For this review, take the finished solid that the model builds, in its own axes (mm). Face numbers are marked on the shaded views. A direction names the side the tool comes from. Round coordinates to 2 decimals unless told otherwise and drop trailing zeros. Order: outer loops, then holes, each group sorted by start corner. A loop starts at its lowest first (then second) coordinate and runs counter-clockwise, first axis right, second up. Notation, with made-up numbers: (-3.5, 54) -> (14.5, 54) arc R6 ccw to (14.5, 60) -> close; hole circle Ø1 at (12, 80.5). An arc over 180 degrees is marked (long way). Answer in a Markdown table with one row per item.
```python
from build123d import *

# Parameters (mm, degrees)
SKETCH1_W           = 300
SKETCH1_H           = 300
BOSS_EXTRUDE1_DEPTH = 120
SKETCH3_R           = 17.5
BOSS_EXTRUDE3_DEPTH = 60
FILLET1_R           = 5
SKETCH4_R           = 51
BOSS_EXTRUDE4_DEPTH = 50
FILLET2_R           = 50
SKETCH6_R           = 7.5
BOSS_EXTRUDE5_DEPTH = 20


with BuildPart() as part:
    # Sketch1 → Boss-Extrude1 (new body)
    with BuildSketch(Plane(origin=(0, 0, 0), x_dir=(1, 0, 0), z_dir=(0, 1, 0))):
        Rectangle(SKETCH1_W, SKETCH1_H)
    extrude(amount=BOSS_EXTRUDE1_DEPTH)

    # Sketch3 → Boss-Extrude3 (add)
    with BuildSketch(Plane.XY.offset(150)):
        with Locations(Location((-115, 25, 0), (0, 0, 180))):
            Circle(SKETCH3_R)
    boss_extrude3 = extrude(amount=BOSS_EXTRUDE3_DEPTH)

    # Mirror1: Boss-Extrude3 across plane
    add(boss_extrude3.mirror(Plane.XY))

    # Fillet1
    fillet1_edges = [part.edges().sort_by_distance(p)[0] for p in [
        (-97.5, 25, 150),
        (-97.5, 25, -150),
    ]]
    fillet(fillet1_edges, radius=FILLET1_R)

    # Sketch4 → Boss-Extrude4 (add)
    with BuildSketch(Plane.XZ):
        with Locations(Location((90, 0, 0), (0, 0, 90))):
            Circle(SKETCH4_R)
    extrude(amount=BOSS_EXTRUDE4_DEPTH)

    # Fillet2
    fillet2_edges = [part.edges().sort_by_distance(p)[0] for p in [
        (90, -50, -51),
    ]]
    fillet(fillet2_edges, radius=FILLET2_R - 0.0001)  # a hair under: the kernel refuses the full size

    # Sketch6 → Boss-Extrude5 (add)
    with BuildSketch(Plane(origin=(150, 0, 0), x_dir=(0, 0, -1), z_dir=(1, 0, 0))):
        with Locations(Location((-75, 50, 0), (0, 0, 180))):
            Circle(SKETCH6_R)
        with Locations(Location((75, 50, 0), (0, 0, 180))):
            Circle(SKETCH6_R)
    extrude(amount=BOSS_EXTRUDE5_DEPTH)


solid = part.part
```
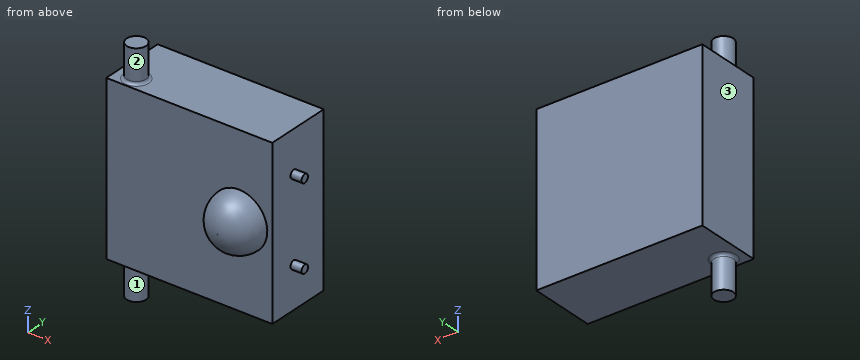
Q1. Take a section at A-A, the plane z = -75. Write out the cut boundary in (x, y).
Answer key:
| item | result |
|---|---|
| outline | (-150, 0) -> (150, 0) -> (150, 42.5) -> (170, 42.5) -> (170, 57.5) -> (150, 57.5) -> (150, 120) -> (-150, 120) -> close |
Q2. Take a section at B-B, the plane x = -115. Write out the cut boundary in (y, z), then the cut area to 3 significant figures.
Answer key:
| item | result |
|---|---|
| outline | (0, -150) -> (2.5, -150) arc R5 cw to (7.5, -155) -> (7.5, -210) -> (42.5, -210) -> (42.5, -155) arc R5 cw to (47.5, -150) -> (120, -150) -> (120, 150) -> (47.5, 150) arc R5 cw to (42.5, 155) -> (42.5, 210) -> (7.5, 210) -> (7.5, 155) arc R5 cw to (2.5, 150) -> (0, 150) -> close |
| area | 40,200 mm^2 |
Q3. Clearance check with flat-ended pins moving along their axes: pin 1 Ø3 at (x, y) = (-26, 53.5) entering from +Z; pin 2 Ø4 at (y, z) = (34, -102.5) entering from +X; pin 3 Ø3 at (x, z) = (-7.5, 92.5) entering from -Y. State where each tip first meets the part, or that it passes through.
Answer key:
| item | result |
|---|---|
| pin 1 | stops at z = 150 |
| pin 2 | stops at x = 150 |
| pin 3 | stops at y = 0 |
Q4. Take a section at C-C, the plane y = 67. Write out the cut boundary in (x, z), then the cut area to 3 significant figures.
Answer key:
| item | result |
|---|---|
| outline | (-150, -150) -> (150, -150) -> (150, 150) -> (-150, 150) -> close |
| area | 90,000 mm^2 |
Q5. Take a section at D-D, the plane x = -66.5. Write out the cut boundary in (y, z).
Answer key:
| item | result |
|---|---|
| outline | (0, -150) -> (120, -150) -> (120, 150) -> (0, 150) -> close |
Q6. Tool access review of the marked faces 1, 2 and 3: name each direction out of +Z, -Z, +X, -X, +Y, -Y from which nothing blocks a thin tool from reaching the whole face with its end or side.
Answer key:
| item | result |
|---|---|
| face 1 | -Z |
| face 2 | +Z |
| face 3 | +Z, -Z, -X, +Y, -Y |
Q7. To check wall thickness, follow probe 1 along X at (y, z) = (21.5, -99.5); probe 2 along Y at (x, z) = (-131.5, 111). State the ranges of each line that lie inside material, in increasing order.
Answer key:
| item | result |
|---|---|
| probe 1 | x = -150 to 150 |
| probe 2 | y = 0 to 120 |
